Work out the finished part from the listing and answer in its coordinate system (mm). Face numbers are marked on the shaded views. A direction names the side the tool comes from. Round coordinates to 2 decimals unless told otherwise and drop trailing zeros. Order: outer loops, then holes, each group sorted by start corner. A loop starts at its lowest first (then second) coordinate and runs counter-clockwise, first axis right, second up. Notation, with made-up numbers: (36.5, 62.5) - (40.5, 62.5) arc R16 ccw to (40.5, 80.5) - close; hole circle Ø5 at (5.5, -34). An arc over 180 degrees is marked (long way). Use one line per item in the form item = value. Start each with the question number.
Q1. Which of the six approach directions +Z, -Z, +X, -X, +Y, -Y give full straight-line access (tool end or side, diameter ignored) to the marked faces 5, 6 and 7?
Q2. The part is cut by section C-C on y = 17.5. Determine the outline of the cut face in (x, z), plus the area to 3 significant figures.
Q3. The part is cut by section D-D on z = 5.25. Determine the outline of the cut face in (x, y), plus the area to 3 significant figures.
Q4. Given P1, Ø8, axis at x = -17.5, y = -6, coming from the +Z side; P2, Ø8, axis at y = 11, z = 15.5, coming from the +X side; P3, Ø3, axis at y = -18.5, z = 5, coming from the +X side, each flat-ended and moving along its own axis, determine where each tip first touches the part or whether it passes through.
Q5. The part is cut by section B-B on y = 10.5. Determine the outline of the cut face in (x, z), plus the area to 3 significant figures.
Q6. For a pull along X with two mould halves and no side action, classify the marked faces 1, 2, 3 and 4 as +X half, -X half, draft (parallel to the pull), parting line (faces both ways), or undercut.
Q7. Find the intervals of material crossed by line 1 (X direction, y = -4, z = 15.75); line 2 (Z direction, x = -24, y = 20.5); line 3 (Y direction, x = 5, z = 15.75), in increasing order. Write a range as [from, to].
Q8. The part is cut by section A-A on x = -2. Determine the outline of the cut face in (y, z).
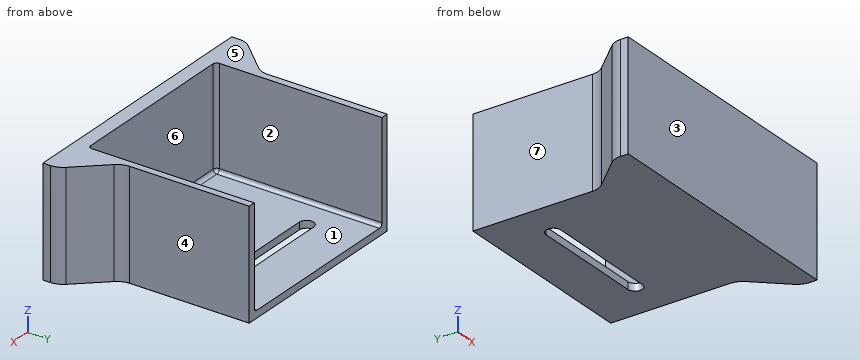
from build123d import *

# Parameters (mm, degrees)
F0_W     = 54
F0_H     = 50
F1_DEPTH = 30
F2_W     = 50
F2_H     = 46
F3_DEPTH = 28
F5_DEPTH = 30
F7_DEPTH = 30.001
F8_R     = 5
F9_R     = 1
F10_R    = 1


with BuildPart() as f1:
    # F0 (on Top) → F1 (new body)
    with BuildSketch(Plane.XY):
        Rectangle(F0_W, F0_H)
    extrude(amount=F1_DEPTH)

    # F2 (on face) → F3 (cut)
    with BuildSketch(Plane.XY.offset(30)):
        with Locations((0, 2)):
            Rectangle(F2_W, F2_H)
    extrude(amount=-F3_DEPTH, mode=Mode.SUBTRACT)

    # F4 (on face) → F5 (join, through all)
    with BuildSketch(Plane.XY.offset(30)):
        Polygon((-37, -25), (-27, -25), (-27, -10), (-37, -21), align=None)
        Polygon((27, -25), (37, -25), (37, -21), (27, -10), align=None)
    extrude(amount=-F5_DEPTH)

    # F6 (on face) → F7 (cut, through all)
    with BuildSketch(Plane(origin=(0, 0, 0), x_dir=(1, 0, 0), z_dir=(0, 0, -1))):
        with BuildLine():
            ThreePointArc((-16, -8.5), (-18, -10.5), (-16, -12.5))
            Line((-16, -12.5), (16, -12.5))
            ThreePointArc((16, -12.5), (18, -10.5), (16, -8.5))
            Line((16, -8.5), (-16, -8.5))
        make_face()
    extrude(amount=-F7_DEPTH, mode=Mode.SUBTRACT)

    # F8
    f8_edges = [f1.edges().sort_by_distance(p)[0] for p in [
        (-27, -10, 15),
        (-37, -21, 15),
        (27, -10, 15),
        (37, -21, 15),
    ]]
    fillet(f8_edges, radius=F8_R)

    # F9
    f9_edges = [f1.edges().sort_by_distance(p)[0] for p in [
        (-25, 2, 2),
        (25, 2, 2),
    ]]
    fillet(f9_edges, radius=F9_R)

    # F10
    f10_edges = [f1.edges().sort_by_distance(p)[0] for p in [
        (-25, -21, 16.5),
    ]]
    fillet(f10_edges, radius=F10_R)


solid = f1.part
Found:
q1.face_5 = +Z, +X, -X, +Y, -Y
q1.face_6 = +Z, +Y
q1.face_7 = +Z, -Z, -X, +Y
q2.outline = (-27, 0) - (27, 0) - (27, 30) - (25, 30) - (25, 3) arc R1 cw to (24, 2) - (-24, 2) arc R1 cw to (-25, 3) - (-25, 30) - (-27, 30) - close
q2.area = 220 mm²
q3.outline = (-37, -25) - (37, -25) - (37, -22.93) arc R5 ccw to (35.7, -19.57) - (28.3, -11.43) arc R5 cw to (27, -8.07) - (27, 25) - (25, 25) - (25, -20) arc R1 cw to (24, -21) - (-24, -21) arc R1 cw to (-25, -20) - (-25, 25) - (-27, 25) - (-27, -8.07) arc R5 cw to (-28.3, -11.43) - (-35.7, -19.57) arc R5 ccw to (-37, -22.93) - close
q3.area = 590 mm²
q4.P1 = 2
q4.P2 = 27
q4.P3 = 36.05
q5.outline = (-27, 0) - (-18, 0) - (-18, 2) - (-24, 2) arc R1 cw to (-25, 3) - (-25, 30) - (-27, 30) - close; (18, 0) - (27, 0) - (27, 30) - (25, 30) - (25, 3) arc R1 cw to (24, 2) - (18, 2) - close
q5.area = 148 mm²
q6.face_1 = undercut
q6.face_2 = undercut
q6.face_3 = draft
q6.face_4 = +X half
q7.line_1 = [-27, -25], [25, 27]
q7.line_2 = [0, 2]
q7.line_3 = [-25, -21]
q8.outline = (-25, 0) - (8.5, 0) - (8.5, 2) - (-20, 2) arc R1 cw to (-21, 3) - (-21, 30) - (-25, 30) - close; (12.5, 0) - (25, 0) - (25, 2) - (12.5, 2) - close
